Geometry check sheet. Reference: drawing and pictorial views, mm from the part's lowest x, y, z. Round coordinates to 2 decimals unless told otherwise and drop trailing zeros. Loops run counter-clockwise (first coordinate to the right, second up) from the corner with the lowest first, then second, coordinate; pieces in that order, holes last. Notation, with made-up numbers: (56.25, 15) -> (62.25, 15) arc R29 ccw to (62.25, 51) -> close; hole circle Ø1 at (19, -21.5). An arc over 180 degrees is marked (long way). Use one line per item in the form item = value. Start each with the question number.
(1) Sectioned sample at B-B (x = 85). Record the cut outline in (y, z) (1 decimal).
(2) Draft check along X on the marked faces 1, 2 and 3. Enter one of: released by +X, released by -X, zero draft, split by the parting line, or undercut.
(3) Go/stop test with flat-tipped pins: pin 1 (23 mm diameter, centred on x = 28.575, y = 28.575, fed in from -Z); pin 2 (4 mm diameter, centred on y = 20, z = 11, fed in from -X); pin 3 (1 mm diameter, centred on y = 8.5, z = 10.5, fed in from -X); pin 4 (1.5 mm diameter, centred on x = 45.5, z = 26, fed in from +Y). Record where each tip stops, or that it passes through.
(4) Sectioned sample at A-A (z = 2.5). State how many separate pieces and enclosed holes the cut face has, and give its area (3 significant figures).
(5) Material ranges on probe 1 along X at (y, z) = (22.5, 15) (1 decimal); probe 2 along Z at (x, y) = (73.5, 39.5); probe 3 along X at (y, z) = (19.5, 30), recorded low to high. Write a range as [from, to].
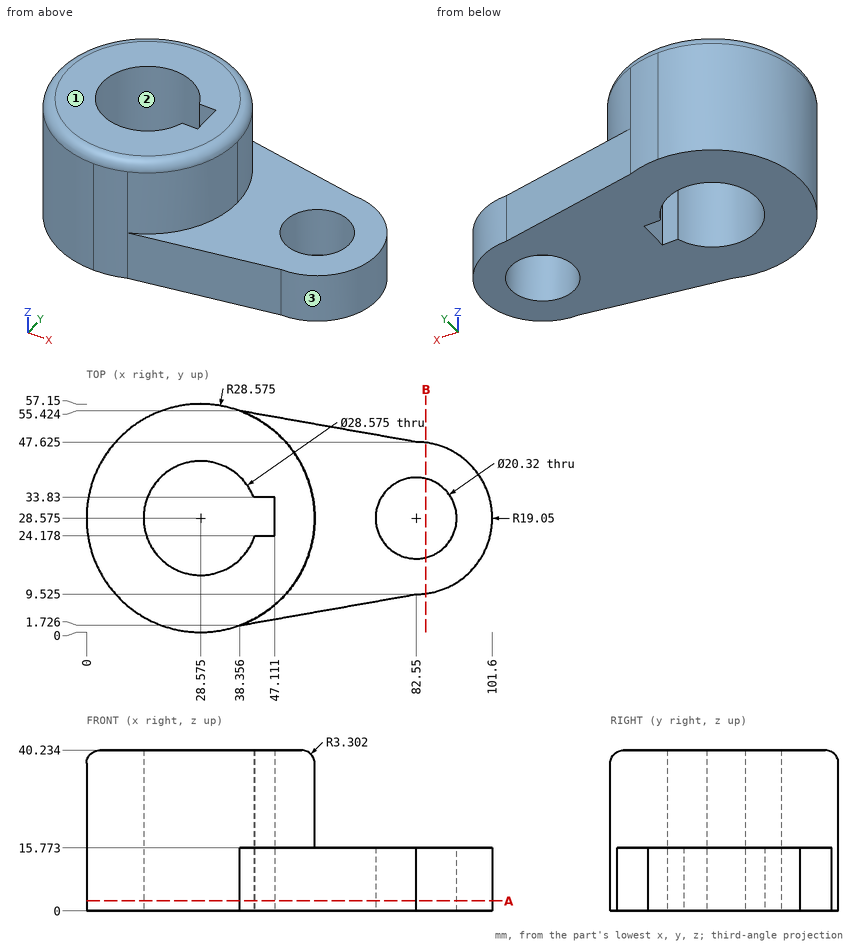
Checks:
q1.outline = (9.7, 0) -> (18.7, 0) -> (18.7, 15.8) -> (9.7, 15.8) -> close; (38.4, 0) -> (47.5, 0) -> (47.5, 15.8) -> (38.4, 15.8) -> close
q2.face_1 = zero draft
q2.face_2 = undercut
q2.face_3 = released by +X
q3.pin_1 = through
q3.pin_2 = 0.77
q3.pin_3 = 7.76
q3.pin_4 = 52.13
q4.separate_pieces = 1
q4.enclosed_holes = 2
q4.area = 3,420 mm2
q5.probe_1 = [0.7, 15.6], [41.5, 74.4], [90.7, 100.6]
q5.probe_2 = [0, 15.77]
q5.probe_3 = [1.48, 17.54], [39.61, 55.67]
